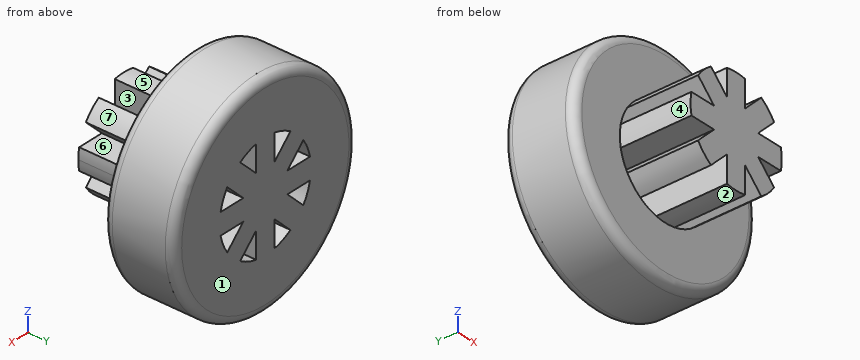
from build123d import *

# Parameters (mm, degrees)
F1_DEPTH = 20
F0_R     = 30
F2_DEPTH = 20
F3_R     = 2.5


with BuildPart() as f1:
    # F0 (on Front) → F1 (new body)
    with BuildSketch(Plane.XZ):
        with BuildLine():
            ThreePointArc((14.6969384567, -3), (14.9240422951, -1.5076344301), (15, 0))
            ThreePointArc((15, 0), (14.9240422951, 1.5076344301), (14.6969384567, 3))
            Line((14.6969384567, 3), (7.2426406871, 3))
            Line((7.2426406871, 3), (12.513625189, 8.2709845019))
            ThreePointArc((12.513625189, 8.2709845019), (10.6066017178, 10.6066017178), (8.2709845019, 12.513625189))
            Line((8.2709845019, 12.513625189), (3, 7.2426406871))
            Line((3, 7.2426406871), (3, 14.6969384567))
            ThreePointArc((3, 14.6969384567), (0, 15), (-3, 14.6969384567))
            Line((-3, 14.6969384567), (-3, 7.2426406871))
            Line((-3, 7.2426406871), (-8.2709845019, 12.513625189))
            ThreePointArc((-8.2709845019, 12.513625189), (-10.6066017178, 10.6066017178), (-12.513625189, 8.2709845019))
            Line((-12.513625189, 8.2709845019), (-7.2426406871, 3))
            Line((-7.2426406871, 3), (-14.6969384567, 3))
            ThreePointArc((-14.6969384567, 3), (-15, 0), (-14.6969384567, -3))
            Line((-14.6969384567, -3), (-7.2426406871, -3))
            Line((-7.2426406871, -3), (-12.513625189, -8.2709845019))
            ThreePointArc((-12.513625189, -8.2709845019), (-10.6066017178, -10.6066017178), (-8.2709845019, -12.513625189))
            Line((-8.2709845019, -12.513625189), (-3, -7.2426406871))
            Line((-3, -7.2426406871), (-3, -14.6969384567))
            ThreePointArc((-3, -14.6969384567), (0, -15), (3, -14.6969384567))
            Line((3, -14.6969384567), (3, -7.2426406871))
            Line((3, -7.2426406871), (8.2709845019, -12.513625189))
            ThreePointArc((8.2709845019, -12.513625189), (10.6066017178, -10.6066017178), (12.513625189, -8.2709845019))
            Line((12.513625189, -8.2709845019), (7.2426406871, -3))
            Line((7.2426406871, -3), (14.6969384567, -3))
        make_face()
    extrude(amount=F1_DEPTH)

    # F0 (on Front) + F1_face (on face) → F2 (join)
    with BuildSketch(Plane.XZ):
        Circle(F0_R)
        with BuildLine():
            ThreePointArc((14.6969384567, 3), (14.9240422951, 1.5076344301), (15, 0))
            ThreePointArc((15, 0), (14.9240422951, -1.5076344301), (14.6969384567, -3))
            ThreePointArc((14.6969384567, -3), (13.8581929877, -5.7402514855), (12.513625189, -8.2709845019))
            ThreePointArc((12.513625189, -8.2709845019), (10.6066017178, -10.6066017178), (8.2709845019, -12.513625189))
            ThreePointArc((8.2709845019, -12.513625189), (5.7402514855, -13.8581929877), (3, -14.6969384567))
            ThreePointArc((3, -14.6969384567), (0, -15), (-3, -14.6969384567))
            ThreePointArc((-3, -14.6969384567), (-5.7402514855, -13.8581929877), (-8.2709845019, -12.513625189))
            ThreePointArc((-8.2709845019, -12.513625189), (-10.6066017178, -10.6066017178), (-12.513625189, -8.2709845019))
            ThreePointArc((-12.513625189, -8.2709845019), (-13.8581929877, -5.7402514855), (-14.6969384567, -3))
            ThreePointArc((-14.6969384567, -3), (-15, 0), (-14.6969384567, 3))
            ThreePointArc((-14.6969384567, 3), (-13.8581929877, 5.7402514855), (-12.513625189, 8.2709845019))
            ThreePointArc((-12.513625189, 8.2709845019), (-10.6066017178, 10.6066017178), (-8.2709845019, 12.513625189))
            ThreePointArc((-8.2709845019, 12.513625189), (-5.7402514855, 13.8581929877), (-3, 14.6969384567))
            ThreePointArc((-3, 14.6969384567), (0, 15), (3, 14.6969384567))
            ThreePointArc((3, 14.6969384567), (5.7402514855, 13.8581929877), (8.2709845019, 12.513625189))
            ThreePointArc((8.2709845019, 12.513625189), (10.6066017178, 10.6066017178), (12.513625189, 8.2709845019))
            ThreePointArc((12.513625189, 8.2709845019), (13.8581929877, 5.7402514855), (14.6969384567, 3))
        make_face(mode=Mode.SUBTRACT)
    with BuildSketch(Plane(origin=(0, 0, 0), x_dir=(1, 0, 0), z_dir=(0, 1, 0))):
        with BuildLine():
            Line((7.2426406871, 3), (12.513625189, 8.2709845019))
            ThreePointArc((12.513625189, 8.2709845019), (10.6066017178, 10.6066017178), (8.2709845019, 12.513625189))
            Line((8.2709845019, 12.513625189), (3, 7.2426406871))
            Line((3, 7.2426406871), (3, 14.6969384567))
            ThreePointArc((3, 14.6969384567), (0, 15), (-3, 14.6969384567))
            Line((-3, 14.6969384567), (-3, 7.2426406871))
            Line((-3, 7.2426406871), (-8.2709845019, 12.513625189))
            ThreePointArc((-8.2709845019, 12.513625189), (-10.6066017178, 10.6066017178), (-12.513625189, 8.2709845019))
            Line((-12.513625189, 8.2709845019), (-7.2426406871, 3))
            Line((-7.2426406871, 3), (-14.6969384567, 3))
            ThreePointArc((-14.6969384567, 3), (-15, 0), (-14.6969384567, -3))
            Line((-14.6969384567, -3), (-7.2426406871, -3))
            Line((-7.2426406871, -3), (-12.513625189, -8.2709845019))
            ThreePointArc((-12.513625189, -8.2709845019), (-10.6066017178, -10.6066017178), (-8.2709845019, -12.513625189))
            Line((-8.2709845019, -12.513625189), (-3, -7.2426406871))
            Line((-3, -7.2426406871), (-3, -14.6969384567))
            ThreePointArc((-3, -14.6969384567), (0, -15), (3, -14.6969384567))
            Line((3, -14.6969384567), (3, -7.2426406871))
            Line((3, -7.2426406871), (8.2709845019, -12.513625189))
            ThreePointArc((8.2709845019, -12.513625189), (10.6066017178, -10.6066017178), (12.513625189, -8.2709845019))
            Line((12.513625189, -8.2709845019), (7.2426406871, -3))
            Line((7.2426406871, -3), (14.6969384567, -3))
            ThreePointArc((14.6969384567, -3), (15, 0), (14.6969384567, 3))
            Line((14.6969384567, 3), (7.2426406871, 3))
        make_face()
    extrude(amount=-F2_DEPTH, dir=(0, -1, 0))

    # F3
    f3_edges = [f1.edges().sort_by_distance(p)[0] for p in [
        (-30, 0, 0),
        (-30, 20, 0),
    ]]
    fillet(f3_edges, radius=F3_R)


solid = f1.part
The listing builds one solid part. Answer for the finished solid, in the listing's coordinates (mm). Face numbers are marked on the shaded views. A direction names the side the tool comes from. Round coordinates to 2 decimals unless told otherwise and drop trailing zeros. Loops run counter-clockwise (first coordinate to the right, second up) from the corner with the lowest first, then second, coordinate; pieces in that order, holes last. Notation, with made-up numbers: M 16,26.25 L 74,26.25 A34 ccw 74,61.25 Z; hole C -24.75,-6.5 d7. An arc over 180 degrees is marked long. Return JSON: item names as keys, results as strings.
Q1. Find the intervals of material crossed by line 1 along Z through (x, y) = (-12, 10); line 2 along Z through (x, y) = (-9, 5); line 3 along Y through (x, z) = (-21, 9), in increasing order. Write a range as from..to.
Results list:
{"line 1": "z = -27.5..-7.76, -3..3, 7.76..27.5", "line 2": "z = -28.62..-4.76, -3..3, 4.76..28.62", "line 3": "y = 0..20"}
Q2. Which of the six approach directions +Z, -Z, +X, -X, +Y, -Y give full straight-line access (tool end or side, diameter ignored) to the marked faces 4, 5, 6 and 7?
Results list:
{"face 4": "-X, -Y", "face 5": "+Z, -Y", "face 6": "+Y, -Y", "face 7": "+Z, +X, -Y"}
Q3. The mould has two halves that part along X. Classify the marked faces 1, 2 and 3: released by +X, released by -X, zero draft, split by the parting line, or undercut.
Results list:
{"face 1": "zero draft", "face 2": "split by the parting line", "face 3": "undercut"}
Q4. Each of these flat-tipped pins is pushed along its axis until it touches: pin 1 Ø2 at (y, z) = (-8.5, -12) entering from -X; pin 2 Ø4 at (y, z) = (13, -21) entering from +X; pin 3 Ø6 at (x, z) = (-5.5, 19) entering from -Y; pin 4 Ø4 at (y, z) = (-5.5, 18) entering from -X (1 decimal). Where does it stop, or does it pass through?
Results list:
{"pin 1": "stops at x = -10.2", "pin 2": "stops at x = 23.22", "pin 3": "stops at y = 0", "pin 4": "passes through"}
Q5. Find section B-B, the plane x = 0. Determine the outline of the cut face in (y, z).
Results list:
{"outline": "M -20,-15 L 0,-15 L 0,-27.5 A2.5 ccw 2.5,-30 L 17.5,-30 A2.5 ccw 20,-27.5 L 20,27.5 A2.5 ccw 17.5,30 L 2.5,30 A2.5 ccw 0,27.5 L 0,15 L -20,15 Z"}
Q6. Find section A-A, the plane y = 12.5. State how many separate pieces and enclosed holes the cut face has, plus the area to 3 significant figures.
Results list:
{"separate pieces": "1", "enclosed holes": "8", "area": "2,660 mm2"}
